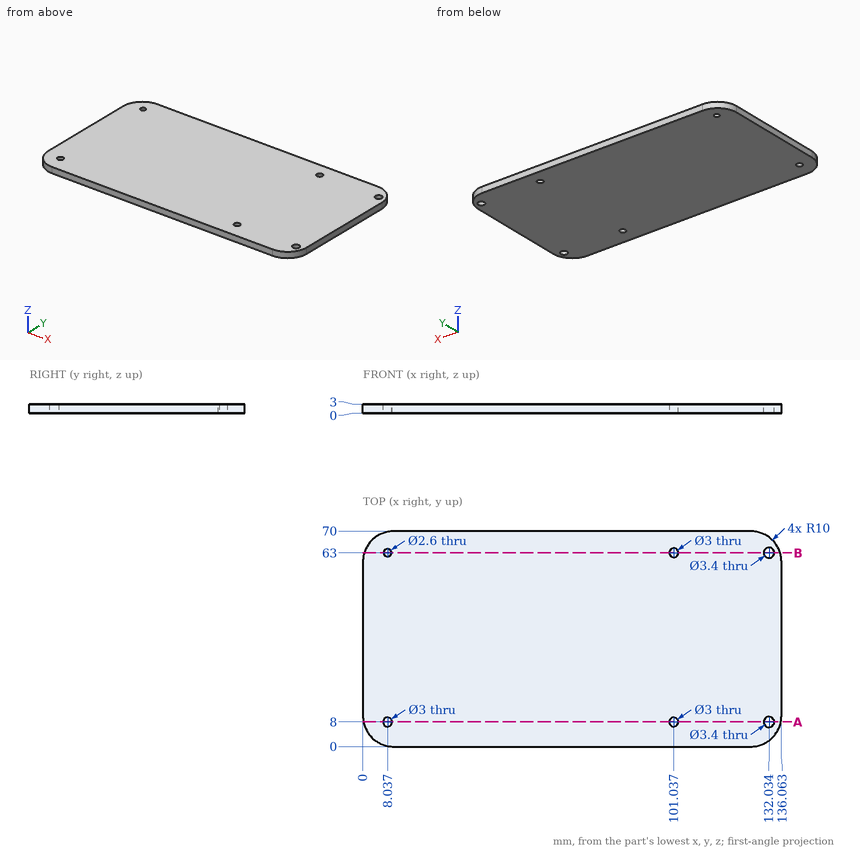
Print and shaded views of the part. All mm, measured from the part's lowest x, y and z. Give positions to 0.01 mm unless a question says otherwise; leave off trailing zeros. Loops run counter-clockwise (first coordinate to the right, second up) from the corner with the lowest first, then second, coordinate; pieces in that order, holes last.
1) Wall check: line 1 (Y direction, x = 126.5, z = 0.2); line 2 (X direction, y = 60.5, z = 2.5). Give the ranges that are in metal, low to high.
2) Saw through at B-B (y = 63). Write the cut outline in (x, z).
3) Saw through at A-A (y = 8). Write the cut outline in (x, z), plus the area to 3 significant figures.
4) Flat gauge pin, fed straight in: pin 1 Ø2 at (x, y) = (132.03, 63) entering from +Z. Where does the tip first touch, or does it go through?
Answer block:
1. line 1: y = 0.01 to 69.99
1. line 2: x = 0.01 to 136.05
2. outline: (0.46, 0) - (6.74, 0) - (6.74, 3) - (0.46, 3) - close; (9.34, 0) - (99.54, 0) - (99.54, 3) - (9.34, 3) - close; (102.54, 0) - (130.33, 0) - (130.33, 3) - (102.54, 3) - close; (133.73, 0) - (135.6, 0) - (135.6, 3) - (133.73, 3) - close
3. outline: (0.2, 0) - (6.54, 0) - (6.54, 3) - (0.2, 3) - close; (9.54, 0) - (99.54, 0) - (99.54, 3) - (9.54, 3) - close; (102.54, 0) - (130.33, 0) - (130.33, 3) - (102.54, 3) - close; (133.73, 0) - (135.86, 0) - (135.86, 3) - (133.73, 3) - close
3. area: 379 mm2
4. pin 1: passes through
